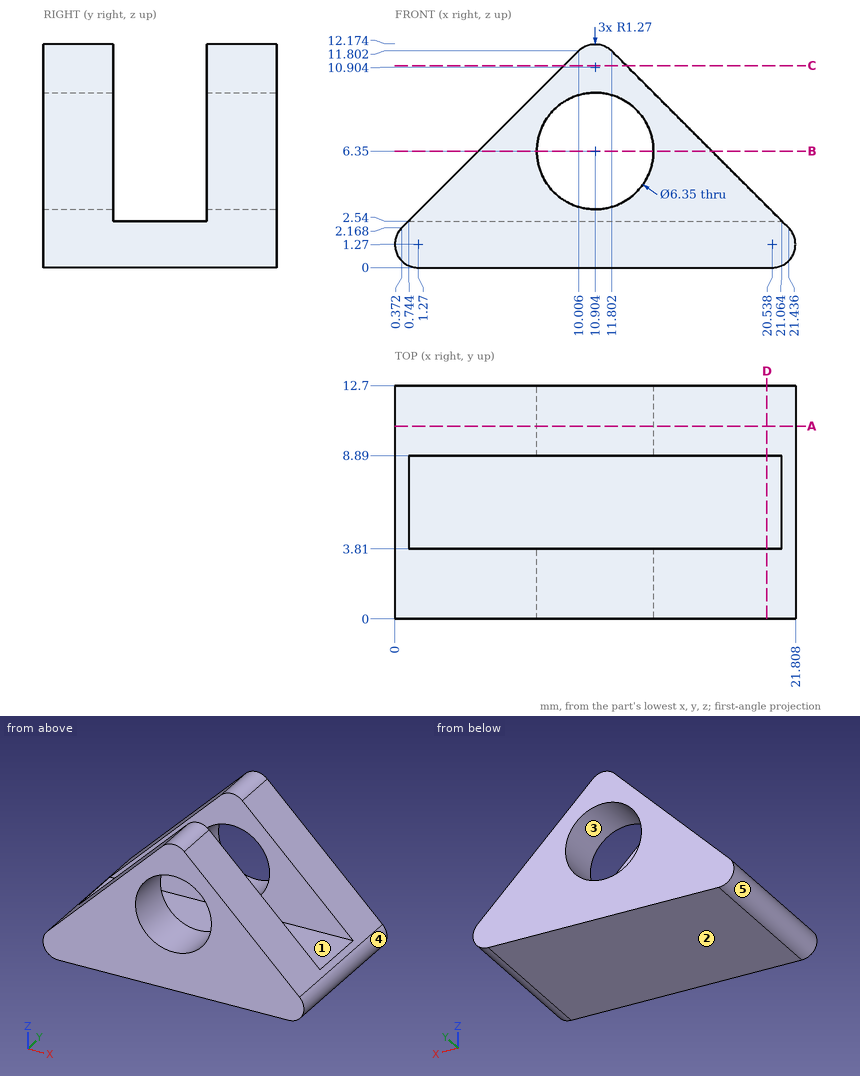
Could you check a few things on this drawing? It's one solid part, dimensions in mm from its lowest x, y, z. A direction names the side the tool comes from. Give positions to 0.01 mm unless a question says otherwise; leave off trailing zeros. Order: outer loops, then holes, each group sorted by start corner. A loop starts at its lowest first (then second) coordinate and runs counter-clockwise, first axis right, second up. Notation, with made-up numbers: (-3.5, -5.5) -> (14.5, -5.5) arc R16 cw to (14.5, 16.5) -> close; hole circle Ø1 at (50, 29.5). An arc over 180 degrees is marked (long way). Use CSV: the item, a comma, the result in double quotes. Start each with the question number.
Item 1: I'm going to push flat-ended pins straight in: P1, Ø5, axis at x = 10, z = 8.5, coming from the +Y side; P2, Ø3, axis at y = 10.5, z = 8.5, coming from the +X side; P3, Ø1.5, axis at x = 6, y = 7, coming from the +Z side; P4, Ø5.5, axis at x = 10.9, z = 6.35, coming from the +Y side (1 decimal). Where does each tip first touch, or does it pass through?
Item 2: Suppose I cut it at B-B (z = 6.35). List the corners of the cut face in (x, y) for me, and give its area (3 significant figures).
Item 3: Suppose I cut it at C-C (z = 11). List the corners of the cut face in (x, y) for me.
Item 4: Suppose I cut it at A-A (y = 10.5). List the corners of the cut face in (x, z) for me (3 decimals), and give its area (3 significant figures).
Item 5: Suppose I cut it at D-D (x = 20.25). List the corners of the cut face in (y, z) for me, and give its area (3 significant figures).
Item 6: On a 3-axis mill with a long thin cutter (end or side, diameter ignored), from which of +Z, -Z, +X, -X, +Y, -Y can I reach the whole of each face in a straight line? I mean the marked faces 1 and 2. Say none if no direction works.
Item 7: If I drill on probe 1 along Y at (x, z) = (7.25, 4.5); probe 2 along Z at (x, y) = (1.25, 4.75); probe 3 along X at (y, z) = (10, 3.5) (1 decimal), over which ranges is the centre line in solid material (lowest first)? Write a range as [from, to].
Item 8: Thinking about a two-plate mould opening in X: for the marked faces 3, 4 and 5, which applies, pulls with the +X half, pulls with the -X half, needs draft (parallel to the pull), parting line crosses it, or undercut?
Answer block:
1,P1,"stops at y = 12.7"
1,P2,"stops at x = 16.6"
1,P3,"stops at z = 2.54"
1,P4,"passes through"
2,outline,"(4.55, 0) -> (7.73, 0) -> (7.73, 3.81) -> (4.55, 3.81) -> close; (4.55, 8.89) -> (7.73, 8.89) -> (7.73, 12.7) -> (4.55, 12.7) -> close; (14.08, 0) -> (17.25, 0) -> (17.25, 3.81) -> (14.08, 3.81) -> close; (14.08, 8.89) -> (17.25, 8.89) -> (17.25, 12.7) -> (14.08, 12.7) -> close"
2,area,"48.4 mm^2"
3,outline,"(9.2, 0) -> (12.6, 0) -> (12.6, 3.81) -> (9.2, 3.81) -> close; (9.2, 8.89) -> (12.6, 8.89) -> (12.6, 12.7) -> (9.2, 12.7) -> close"
4,outline,"(0.372, 2.168) arc R1.27 ccw to (1.27, 0) -> (20.538, 0) arc R1.27 ccw to (21.436, 2.168) -> (11.802, 11.802) arc R1.27 ccw to (10.006, 11.802) -> close; hole circle Ø6.35 at (10.904, 6.35)"
4,area,"125 mm^2"
5,outline,"(0, 0) -> (12.7, 0) -> (12.7, 3.35) -> (8.89, 3.35) -> (8.89, 2.54) -> (3.81, 2.54) -> (3.81, 3.35) -> (0, 3.35) -> close"
5,area,"38.5 mm^2"
6,face 1,"+Z, +X, -X"
6,face 2,"-Z, +X, -X, +Y, -Y"
7,probe 1,"y = [0, 3.81], [8.89, 12.7]"
7,probe 2,"z = [0, 2.54]"
7,probe 3,"x = [1.7, 9.5], [12.3, 20.1]"
8,face 3,"undercut"
8,face 4,"pulls with the +X half"
8,face 5,"pulls with the -X half"
